```python
from build123d import *

# Parameters (mm, degrees)
F0_R     = 1.4
F0_W     = 10
F0_H     = 10
F1_DEPTH = 4.5


with BuildPart() as f1:
    # F0 (on Top) → F1 (new body)
    with BuildSketch(Plane.XY):
        with BuildLine():
            Line((-31.5, -38), (31.5, -38))
            ThreePointArc((31.5, -38), (36.096194, -36.096194), (38, -31.5))
            Line((38, -31.5), (38, 31.5))
            ThreePointArc((38, 31.5), (36.096194, 36.096194), (31.5, 38))
            Line((31.5, 38), (-31.5, 38))
            ThreePointArc((-31.5, 38), (-36.096194, 36.096194), (-38, 31.5))
            Line((-38, 31.5), (-38, -31.5))
            ThreePointArc((-38, -31.5), (-36.096194, -36.096194), (-31.5, -38))
        make_face()
        with Locations((-31, -31)):
            Circle(F0_R, mode=Mode.SUBTRACT)
        with Locations((31, -31)):
            Circle(F0_R, mode=Mode.SUBTRACT)
        with Locations((-31, 31)):
            Circle(F0_R, mode=Mode.SUBTRACT)
        Rectangle(F0_W, F0_H, mode=Mode.SUBTRACT)
        with Locations((31, 31)):
            Circle(F0_R, mode=Mode.SUBTRACT)
    extrude(amount=F1_DEPTH)


solid = f1.part
```
Geometry: final body of the model. Coordinates: model frame, mm. A direction names the side the tool comes from. Coordinates: 2 decimals unless noted, no trailing zeros. Loops run counter-clockwise (first coordinate to the right, second up) from the corner with the lowest first, then second, coordinate; pieces in that order, holes last. Notation, with made-up numbers: (-22.5, -28.5) -> (23.5, -28.5) arc R28 ccw to (23.5, -4.5) -> close; hole circle Ø8 at (-6, -20.75). An arc over 180 degrees is marked (long way). Use a Markdown table: item, result. Add a question column.
(1) Line query: line 1 along Y through (x, z) = (31, 1.2); line 2 along Y through (x, z) = (-2, 2.25). Output: solid intervals per line, ascending.
(2) Mould query, pull axis X, two halves, no side actions, for faces 1 (the cylindrical face through (-36.146, -36.045, 2.218)), 2 (the flat face through (38, 0, 2)), 3 (the flat face through (0, 5, 2)). Classes: pulls with the +X half, pulls with the -X half, needs draft (parallel to the pull), parting line crosses it, or undercut.
(3) Section query A-A, the plane z = 3.05. Return loops of the section in (x, y).
(4) Section query B-B, the plane x = -30.5. Return loops of the section in (y, z), plus the area to 3 significant figures.
(5) Pin query (flat end, axial travel): pin 1 Ø2.5 at (x, y) = (-31, 31) entering from +Z. Return the tip coordinate at first contact, or that it passes through.
(6) Access query for faces 4 (the flat face through (-38, 0, 2)), 5 (the flat face through (5, 0, 2)). Directions: +Z, -Z, +X, -X, +Y, -Y. A direction counts if a zero-diameter tool reaches every point of the face in a straight line with its end or side. Return the directions, or none.
Answer:
| question | item | result |
|---|---|---|
| 1 | line 1 | y = -38 to -32.4, -29.6 to 29.6, 32.4 to 38 |
| 1 | line 2 | y = -38 to -5, 5 to 38 |
| 2 | face 1 | pulls with the -X half |
| 2 | face 2 | pulls with the +X half |
| 2 | face 3 | undercut |
| 3 | outline | (-38, -31.5) arc R6.5 ccw to (-31.5, -38) -> (31.5, -38) arc R6.5 ccw to (38, -31.5) -> (38, 31.5) arc R6.5 ccw to (31.5, 38) -> (-31.5, 38) arc R6.5 ccw to (-38, 31.5) -> close; hole circle Ø2.8 at (-31, -31); hole circle Ø2.8 at (-31, 31); hole (-5, -5) -> (5, -5) -> (5, 5) -> (-5, 5) -> close; hole circle Ø2.8 at (31, -31); hole circle Ø2.8 at (31, 31) |
| 4 | outline | (-38, 0) -> (-32.31, 0) -> (-32.31, 4.5) -> (-38, 4.5) -> close; (-29.69, 0) -> (29.69, 0) -> (29.69, 4.5) -> (-29.69, 4.5) -> close; (32.31, 0) -> (38, 0) -> (38, 4.5) -> (32.31, 4.5) -> close |
| 4 | area | 318 mm^2 |
| 5 | pin 1 | passes through |
| 6 | face 4 | +Z, -Z, -X, +Y, -Y |
| 6 | face 5 | +Z, -Z |
